Source: CAD feature listing. Evaluate the final solid. Frame: model axes, mm. Face numbers are marked on the shaded views. A direction names the side the tool comes from. Round coordinates to 2 decimals unless told otherwise and drop trailing zeros. Write each loop counter-clockwise with the first axis right and the second up, starting at its lowest first coordinate (ties: lowest second). Pieces come first, ordered by that corner, then holes.
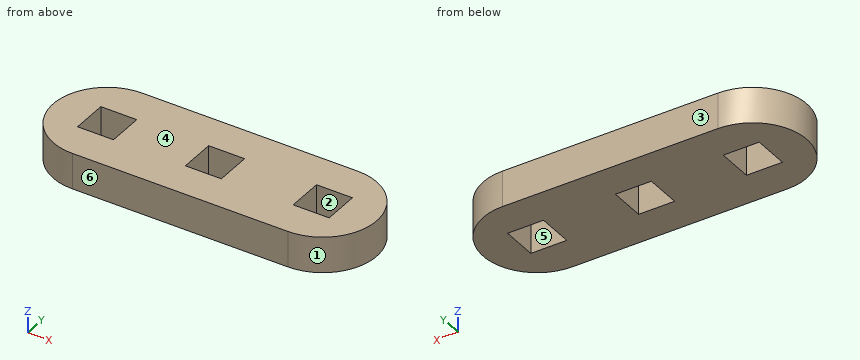
from build123d import *

# Parameters (mm, degrees)
MODEL_W                 = 3
MODEL_H                 = 3
SALIENTE_EXTRUIR1_DEPTH = 3


with BuildPart() as part:
    # Model → Saliente-Extruir1 (new body)
    with BuildSketch(Plane.XY):
        with BuildLine():
            Line((12.437380241, 299.545342772), (30.437380241, 299.545342772))
            ThreePointArc((30.437380241, 299.545342772), (34.937380241, 295.045342772), (30.437380241, 290.545342772))
            Line((30.437380241, 290.545342772), (12.437380241, 290.545342772))
            ThreePointArc((12.437380241, 290.545342772), (7.937380241, 295.045342772), (12.437380241, 299.545342772))
        make_face()
        with Locations((12.437380241, 295.045342772)):
            Rectangle(MODEL_W, MODEL_H, mode=Mode.SUBTRACT)
        with Locations((21.437380241, 295.045342772)):
            Rectangle(MODEL_W, MODEL_H, mode=Mode.SUBTRACT)
        with Locations((30.437380241, 295.045342772)):
            Rectangle(MODEL_W, MODEL_H, mode=Mode.SUBTRACT)
    extrude(amount=SALIENTE_EXTRUIR1_DEPTH)


solid = part.part
1) Section query C-C on y = 295.75. Return the cut outline in (x, z).
Taken from the geometry:
outline: (7.99, 0) - (10.94, 0) - (10.94, 3) - (7.99, 3) - close; (13.94, 0) - (19.94, 0) - (19.94, 3) - (13.94, 3) - close; (22.94, 0) - (28.94, 0) - (28.94, 3) - (22.94, 3) - close; (31.94, 0) - (34.88, 0) - (34.88, 3) - (31.94, 3) - close
2) Section query D-D on x = 12. Return the cut outline in (y, z), then the cut area to 3 significant figures.
Taken from the geometry:
outline: (290.57, 0) - (293.55, 0) - (293.55, 3) - (290.57, 3) - close; (296.55, 0) - (299.52, 0) - (299.52, 3) - (296.55, 3) - close
area: 17.9 mm2
3) Section query A-A on z = 2.25. Return the cut outline in (x, y).
Taken from the geometry:
outline: (12.44, 290.55) - (30.44, 290.55) arc R4.5 ccw to (30.44, 299.55) - (12.44, 299.55) arc R4.5 ccw to start; hole (10.94, 293.55) - (13.94, 293.55) - (13.94, 296.55) - (10.94, 296.55) - close; hole (19.94, 293.55) - (22.94, 293.55) - (22.94, 296.55) - (19.94, 296.55) - close; hole (28.94, 293.55) - (31.94, 293.55) - (31.94, 296.55) - (28.94, 296.55) - close
4) Contact query for a flat-ended pin moving along its axis: P1, Ø0.9, axis at y = 295.5, z = 2, coming from the -X side. Output: stop coordinate, or through.
Taken from the geometry:
P1: stops at x = 7.94
5) Material intervals for line 1 (X direction, y = 295, z = 2.5); line 2 (Y direction, x = 21.5, z = 1.7); line 3 (X direction, y = 294, z = 0.4), sorted ascending.
Taken from the geometry:
line 1: x = 7.94 to 10.94, 13.94 to 19.94, 22.94 to 28.94, 31.94 to 34.94
line 2: y = 290.55 to 293.55, 296.55 to 299.55
line 3: x = 8.06 to 10.94, 13.94 to 19.94, 22.94 to 28.94, 31.94 to 34.81
6) Pull-direction query (Y, two-part tool) for the marked faces 1, 2, 3 and 4; classes: released by +Y, released by -Y, zero draft, split by the parting line, or undercut.
Taken from the geometry:
face 1: split by the parting line
face 2: undercut
face 3: released by +Y
face 4: zero draft
7) Reachability of the marked faces 5 and 6 from +Z, -Z, +X, -X, +Y, -Y: full face, straight path, thin tool, end or side. Return the list, or none.
Taken from the geometry:
face 5: +Z, -Z
face 6: +Z, -Z, +X, -X, -Y
8) Section query B-B on x = 21.75. Return the cut outline in (y, z), then the cut area to 3 significant figures.
Taken from the geometry:
outline: (290.55, 0) - (293.55, 0) - (293.55, 3) - (290.55, 3) - close; (296.55, 0) - (299.55, 0) - (299.55, 3) - (296.55, 3) - close
area: 18.0 mm2
